Design review of the part built by this model. Coordinates are the model's own, in mm. Coordinates: 2 decimals unless noted, no trailing zeros. Loops run counter-clockwise (first coordinate to the right, second up) from the corner with the lowest first, then second, coordinate; pieces in that order, holes last. Notation, with made-up numbers: (-3, 42) -> (17, 42) arc R8 ccw to (17, 57) -> close; hole circle Ø10 at (31, -33). An arc over 180 degrees is marked (long way). Answer as a JSON object with one key per item and string values.
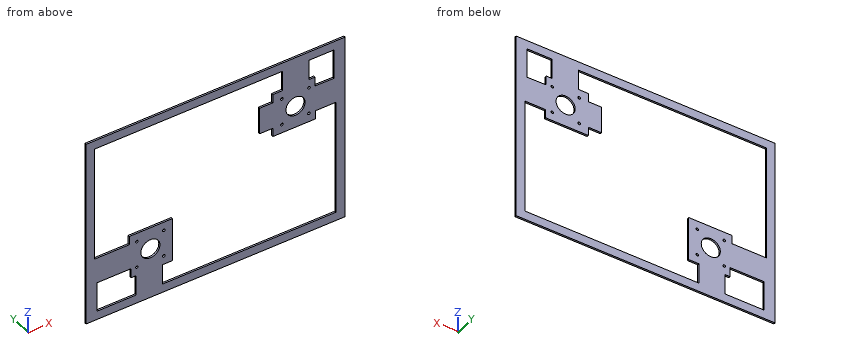
```python
from build123d import *

# Parameters (mm, degrees)
SKETCH1_W           = 218
SKETCH1_H           = 2
BOSS_EXTRUDE1_DEPTH = 298
SKETCH2_R           = 11
SKETCH2_R_2         = 1.5
CUT_EXTRUDE1_DEPTH  = 10


with BuildPart() as part:
    # Sketch1 → Boss-Extrude1 (new body)
    with BuildSketch(Plane(origin=(0, 0, 0), x_dir=(0, 0, -1), z_dir=(1, 0, 0))):
        with Locations((82.3216851, 1)):
            Rectangle(SKETCH1_W, SKETCH1_H)
    extrude(amount=BOSS_EXTRUDE1_DEPTH)

    # Sketch2 → Cut-Extrude1 (cut)
    with BuildSketch(Plane(origin=(0, 2, 0), x_dir=(1, 0, 0), z_dir=(0, 1, 0))):
        with Locations((74, 132.3216851)):
            Circle(SKETCH2_R)
        with Locations((89.5, 116.8216851)):
            Circle(SKETCH2_R_2)
        with Locations((58.5, 116.8216851)):
            Circle(SKETCH2_R_2)
        with Locations((89.5, 147.8216851)):
            Circle(SKETCH2_R_2)
        with Locations((58.5, 147.8216851)):
            Circle(SKETCH2_R_2)
        with Locations((256.33130124, 47.719426297)):
            Circle(SKETCH2_R_2)
        with Locations((256.457517214, 16.719426297)):
            Circle(SKETCH2_R_2)
        with Locations((225.33130124, 16.719426297)):
            Circle(SKETCH2_R_2)
        with Locations((225.33130124, 47.719426297)):
            Circle(SKETCH2_R_2)
        with Locations((240.957517214, 32.219426297)):
            Circle(SKETCH2_R)
        Polygon((12.887616176, 181.3216851), (57.721228679, 181.3216851), (57.721228679, 157.8216851), (51.65209525, 157.8216851), (51.65209525, 146.8216851), (12.887616176, 146.8216851), (12.887616176, 159.517007057), align=None)
        Polygon((149, -16.6783149), (104.471210326, -16.6783149), (10, -16.6783149), (10, 89.941809838), (10, 116.8216851), (49.873323929, 116.8216851), (49.873323929, 106.8216851), (99.5, 106.8216851), (99.5, 157.8216851), (87.721228679, 157.8216851), (87.721228679, 181.3216851), (101.200621078, 181.3216851), (149, 181.3216851), (287.459100292, 181.3216851), (287.459100292, 47.8216851), (263.876177895, 47.8216851), (263.876177895, 57.719426297), (214.790401532, 57.719426297), (214.790401532, 47.719426297), (199.762615123, 47.719426297), (199.762615123, 16.719426297), (214.790401532, 16.719426297), (214.790401532, 6.77711424), (226.154489119, 6.77711424), (226.154489119, -16.6783149), align=None)
        Polygon((285.112383824, -16.6783149), (285.112383824, 5.126363143), (285.112383824, 17.8216851), (263.305421964, 17.488619524), (263.305421964, 6.719426297), (256.695388827, 6.719426297), (256.695388827, -16.6783149), align=None)
    extrude(amount=-CUT_EXTRUDE1_DEPTH, mode=Mode.SUBTRACT)


solid = part.part
```
1) Add section D-D, the plane x = 23. Give the boundary of the cut face in (y, z), and give its area (3 significant figures).
Completed:
{"outline": "(0, -191.32) -> (2, -191.32) -> (2, -181.32) -> (0, -181.32) -> close; (0, -146.82) -> (2, -146.82) -> (2, -116.82) -> (0, -116.82) -> close; (0, 16.68) -> (2, 16.68) -> (2, 26.68) -> (0, 26.68) -> close", "area": "100 mm²"}
2) Wall thickness on probe 1 along X at (y, z) = (0.95, -110); probe 2 along X at (y, z) = (0.75, -56); probe 3 along Z at (x, y) = (22, 0.95): over which ranges is each line inside the solid? List them lowest first.
Completed:
{"probe 1": "0 to 10, 49.87 to 99.5, 287.46 to 298", "probe 2": "0 to 10, 214.79 to 263.88, 287.46 to 298", "probe 3": "-191.32 to -181.32, -146.82 to -116.82, 16.68 to 26.68"}
3) Add section B-B, the plane x = 171.5. Give the boundary of the cut face in (y, z), and give its area (3 significant figures).
Completed:
{"outline": "(0, -191.32) -> (2, -191.32) -> (2, -181.32) -> (0, -181.32) -> close; (0, 16.68) -> (2, 16.68) -> (2, 26.68) -> (0, 26.68) -> close", "area": "40.0 mm²"}
4) Add section A-A, the plane z = 9. Give the boundary of the cut face in (x, y).
Completed:
{"outline": "(0, 0) -> (10, 0) -> (10, 2) -> (0, 2) -> close; (226.15, 0) -> (256.7, 0) -> (256.7, 2) -> (226.15, 2) -> close; (285.11, 0) -> (298, 0) -> (298, 2) -> (285.11, 2) -> close"}
5) Add section C-C, the plane z = -75.5. Give the boundary of the cut face in (x, y).
Completed:
{"outline": "(0, 0) -> (10, 0) -> (10, 2) -> (0, 2) -> close; (287.46, 0) -> (298, 0) -> (298, 2) -> (287.46, 2) -> close"}
